CAD build for the part. Positions are in the model's coordinates, mm. Give positions to 0.01 mm unless a question says otherwise; leave off trailing zeros. Loops run counter-clockwise (first coordinate to the right, second up) from the corner with the lowest first, then second, coordinate; pieces in that order, holes last. Notation, with made-up numbers: (23.5, -30.75) -> (38.5, -30.75) arc R31 ccw to (38.5, 7.25) -> close; hole circle Ø2 at (22.25, -22.5). An arc over 180 degrees is marked (long way). Use one line per item in the form item = value.
```python
from build123d import *

# Parameters (mm, degrees)
F0_R     = 1
F1_DEPTH = 2


with BuildPart() as f1:
    # F0 (on Top) → F1 (new body)
    with BuildSketch(Plane.XY):
        with BuildLine():
            ThreePointArc((29.346194, 39.596192), (29.346194, 44.545939), (24.396447, 44.545939))
            ThreePointArc((24.396447, 44.545939), (-1.12868, 40.571065), (-26.653806, 44.545939))
            ThreePointArc((-26.653806, 44.545939), (-31.603553, 44.545939), (-31.603553, 39.596192))
            ThreePointArc((-31.603553, 39.596192), (-27.62868, -2.428935), (-31.603553, -44.454061))
            ThreePointArc((-31.603553, -44.454061), (-31.603553, -49.403808), (-26.653806, -49.403808))
            ThreePointArc((-26.653806, -49.403808), (-1.12868, -43.428935), (24.396447, -49.403808))
            ThreePointArc((24.396447, -49.403808), (29.346194, -49.403808), (29.346194, -44.454061))
            ThreePointArc((29.346194, -44.454061), (25.37132, -2.428935), (29.346194, 39.596192))
        make_face()
        with Locations((-29.12868, -46.928935)):
            Circle(F0_R, mode=Mode.SUBTRACT)
        with BuildLine():
            Line((-17.12868, -36.171575), (-17.12868, -21.171575))
            ThreePointArc((-17.12868, -21.171575), (-14.12868, -18.171575), (-11.12868, -21.171575))
            Line((-11.12868, -21.171575), (-11.12868, -36.171575))
            ThreePointArc((-11.12868, -36.171575), (-14.12868, -39.171575), (-17.12868, -36.171575))
        make_face(mode=Mode.SUBTRACT)
        with BuildLine():
            Line((-4.12868, -36.171575), (-4.12868, -21.171575))
            ThreePointArc((-4.12868, -21.171575), (-1.12868, -18.171575), (1.87132, -21.171575))
            Line((1.87132, -21.171575), (1.87132, -36.171575))
            ThreePointArc((1.87132, -36.171575), (-1.12868, -39.171575), (-4.12868, -36.171575))
        make_face(mode=Mode.SUBTRACT)
        with BuildLine():
            Line((8.87132, -36.171575), (8.87132, -21.171575))
            ThreePointArc((8.87132, -21.171575), (11.87132, -18.171575), (14.87132, -21.171575))
            Line((14.87132, -21.171575), (14.87132, -36.171575))
            ThreePointArc((14.87132, -36.171575), (11.87132, -39.171575), (8.87132, -36.171575))
        make_face(mode=Mode.SUBTRACT)
        with Locations((26.87132, -46.928935)):
            Circle(F0_R, mode=Mode.SUBTRACT)
        with BuildLine():
            Line((-17.12868, -11.171575), (-17.12868, 8.828425))
            ThreePointArc((-17.12868, 8.828425), (-14.12868, 11.828425), (-11.12868, 8.828425))
            Line((-11.12868, 8.828425), (-11.12868, -11.171575))
            ThreePointArc((-11.12868, -11.171575), (-14.12868, -14.171575), (-17.12868, -11.171575))
        make_face(mode=Mode.SUBTRACT)
        with Locations((-29.12868, 42.071065)):
            Circle(F0_R, mode=Mode.SUBTRACT)
        with BuildLine():
            Line((-17.12868, 18.828425), (-17.12868, 33.828425))
            ThreePointArc((-17.12868, 33.828425), (-14.12868, 36.828425), (-11.12868, 33.828425))
            Line((-11.12868, 33.828425), (-11.12868, 18.828425))
            ThreePointArc((-11.12868, 18.828425), (-14.12868, 15.828425), (-17.12868, 18.828425))
        make_face(mode=Mode.SUBTRACT)
        with BuildLine():
            Line((-4.12868, -11.171575), (-4.12868, 8.828425))
            ThreePointArc((-4.12868, 8.828425), (-1.12868, 11.828425), (1.87132, 8.828425))
            Line((1.87132, 8.828425), (1.87132, -11.171575))
            ThreePointArc((1.87132, -11.171575), (-1.12868, -14.171575), (-4.12868, -11.171575))
        make_face(mode=Mode.SUBTRACT)
        with BuildLine():
            Line((8.87132, -11.171575), (8.87132, 8.828425))
            ThreePointArc((8.87132, 8.828425), (11.87132, 11.828425), (14.87132, 8.828425))
            Line((14.87132, 8.828425), (14.87132, -11.171575))
            ThreePointArc((14.87132, -11.171575), (11.87132, -14.171575), (8.87132, -11.171575))
        make_face(mode=Mode.SUBTRACT)
        with BuildLine():
            Line((-4.12868, 18.828425), (-4.12868, 33.828425))
            ThreePointArc((-4.12868, 33.828425), (-1.12868, 36.828425), (1.87132, 33.828425))
            Line((1.87132, 33.828425), (1.87132, 18.828425))
            ThreePointArc((1.87132, 18.828425), (-1.12868, 15.828425), (-4.12868, 18.828425))
        make_face(mode=Mode.SUBTRACT)
        with BuildLine():
            Line((8.87132, 18.828425), (8.87132, 33.828425))
            ThreePointArc((8.87132, 33.828425), (11.87132, 36.828425), (14.87132, 33.828425))
            Line((14.87132, 33.828425), (14.87132, 18.828425))
            ThreePointArc((14.87132, 18.828425), (11.87132, 15.828425), (8.87132, 18.828425))
        make_face(mode=Mode.SUBTRACT)
        with Locations((26.87132, 42.071065)):
            Circle(F0_R, mode=Mode.SUBTRACT)
    extrude(amount=F1_DEPTH)


solid = f1.part
```
1. Cut at B-B, the plane x = 12. Write the cut outline in (y, z), then the cut area to 3 significant figures.
Result sheet:
outline = (-44.95, 0) -> (-39.17, 0) -> (-39.17, 2) -> (-44.95, 2) -> close; (-18.17, 0) -> (-14.17, 0) -> (-14.17, 2) -> (-18.17, 2) -> close; (11.83, 0) -> (15.83, 0) -> (15.83, 2) -> (11.83, 2) -> close; (36.83, 0) -> (41.6, 0) -> (41.6, 2) -> (36.83, 2) -> close
area = 37.1 mm^2
2. Drop flat-ended pins along their axis: P1, Ø1, axis at y = -31.5, z = 1, coming from the -X side; P2, Ø1, axis at y = -3.5, z = 1.5, coming from the +X side; P3, Ø1, axis at y = 29, z = 1, coming from the -X side. Give the stop position or say it passes through.
Result sheet:
P1 = -29.59
P2 = 25.38
P3 = -29.91
3. Drill centre lines: line 1 (X direction, y = -11, z = 1.7); line 2 (X direction, y = -28, z = 0.2); line 3 (Y direction, x = -1.5, z = 1.05). Where is each one in solid material? Low to high.
Result sheet:
line_1 = -27.79 to -17.13, -11.13 to -4.13, 1.87 to 8.87, 14.87 to 25.54
line_2 = -29.09 to -17.13, -11.13 to -4.13, 1.87 to 8.87, 14.87 to 26.83
line_3 = -43.43 to -39.15, -18.19 to -14.15, 11.81 to 15.85, 36.81 to 40.57
4. Cut at C-C, the plane z = 1.55. State how many separate pieces and enclosed holes the cut face has, then the cut area to 3 significant figures.
Result sheet:
separate_pieces = 1
enclosed_holes = 13
area = 3,800 mm^2
5. Cut at A-A, the plane y = 0. Write the cut outline in (x, z).
Result sheet:
outline = (-27.64, 0) -> (-17.13, 0) -> (-17.13, 2) -> (-27.64, 2) -> close; (-11.13, 0) -> (-4.13, 0) -> (-4.13, 2) -> (-11.13, 2) -> close; (1.87, 0) -> (8.87, 0) -> (8.87, 2) -> (1.87, 2) -> close; (14.87, 0) -> (25.38, 0) -> (25.38, 2) -> (14.87, 2) -> close
6. Mould opens along Y. For faces 1 (the flat face through (5, -2, 0)), 2 (the flat face through (8.871, -1, 1)), 3 (the cylindrical face through (-0.77, 40.57, 0.99)) say: pulls with the +Y half, pulls with the -Y half, needs draft (parallel to the pull), parting line crosses it, or undercut.
Result sheet:
face_1 = needs draft
face_2 = undercut
face_3 = pulls with the +Y half
7. Cut at D-D, the plane x = -24. Write the cut outline in (y, z), then the cut area to 3 significant figures.
Result sheet:
outline = (-48.17, 0) -> (43.75, 0) -> (43.75, 2) -> (-48.17, 2) -> close
area = 184 mm^2
